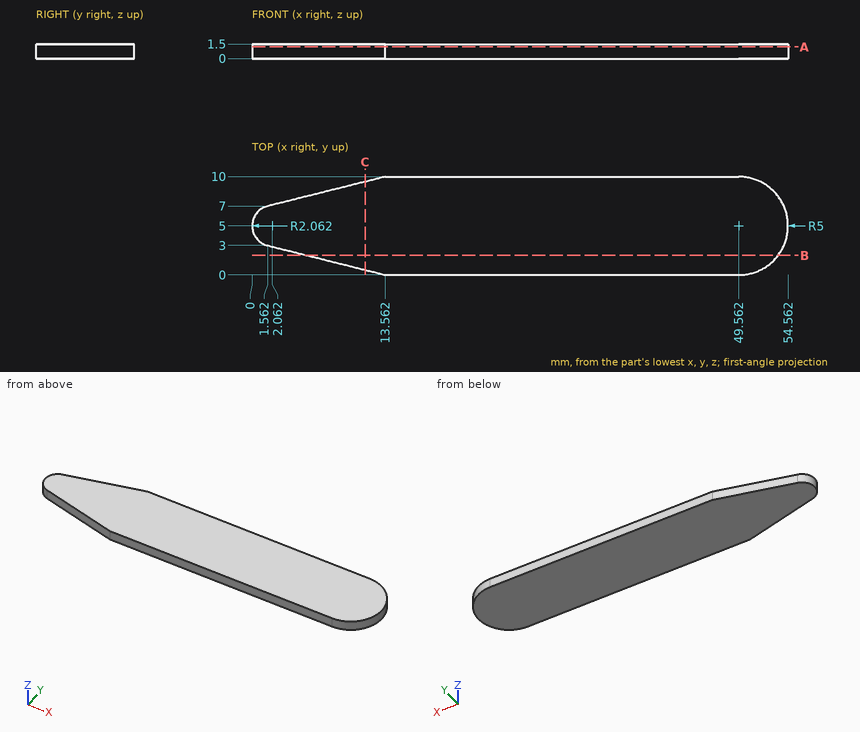
Verification items for this drawing (mm, ordinates from the low corner). Give positions to 0.01 mm unless a question says otherwise; leave off trailing zeros. Write each loop counter-clockwise with the first axis right and the second up, starting at its lowest first coordinate (ties: lowest second). Pieces come first, ordered by that corner, then holes. Notation, with made-up numbers: M 7.5,51.5 L 23.5,51.5 A9 cw 23.5,62.5 Z; hole C 54,87 d5. An arc over 180 degrees is marked long. Use one line per item in the form item = value.
(1) Section check B-B on y = 2. Record the boundary of the cut face in (x, z).
Answer block:
outline = M 5.56,0 L 53.56,0 L 53.56,1.5 L 5.56,1.5 Z
(2) Section check C-C on x = 11.5. Record the boundary of the cut face in (y, z) (1 decimal).
Answer block:
outline = M 0.5,0 L 9.5,0 L 9.5,1.5 L 0.5,1.5 Z
(3) Section check A-A on z = 1.2. Record the boundary of the cut face in (x, y).
Answer block:
outline = M 1.56,3 L 13.56,0 L 49.56,0 A5 ccw 49.56,10 L 13.56,10 L 1.56,7 A2.06 ccw Z
(4) Material ranges on line 1 along Y through (x, z) = (11.5, 0.1) (1 decimal); line 2 along X through (y, z) = (4.5, 0.9); line 3 along Y through (x, z) = (6.5, 0.65) (1 decimal), recorded low to high.
Answer block:
line_1 = 0.5 to 9.5
line_2 = 0.06 to 54.54
line_3 = 1.8 to 8.2
